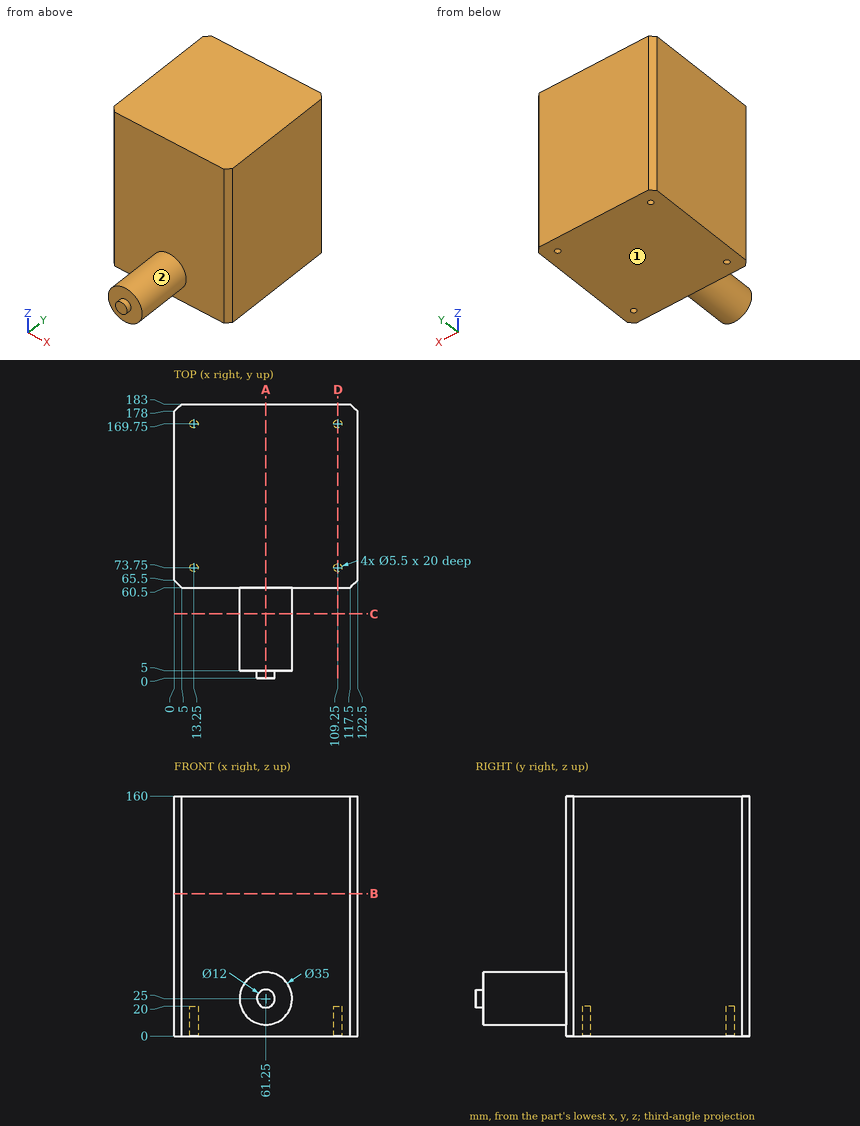
Can you work these out from the drawing? Everything is in mm from the part's minimum corner. A direction names the side the tool comes from. Round coordinates to 2 decimals unless told otherwise and drop trailing zeros. Loops run counter-clockwise (first coordinate to the right, second up) from the corner with the lowest first, then second, coordinate; pieces in that order, holes last. Notation, with made-up numbers: (31, -32) -> (55, -32) arc R29 cw to (55, -2) -> close; hole circle Ø7 at (9, -34). An arc over 180 degrees is marked (long way). Use CSV: the item, a comma, the result in double quotes.
(1) Suppose I cut it at C-C on y = 43. Write out the boundary of the cut face in (x, z), plus the area to 3 significant figures.
Return value:
outline,"circle Ø35 at (61.25, 25)"
area,"962 mm²"
(2) If I drill on probe 1 along Y at (x, z) = (13.25, 5.5); probe 2 along X at (y, z) = (169.75, 7.5); probe 3 along Y at (x, z) = (100.5, 55.5), over which ranges is the centre line in solid material (lowest first)? Write a range as [from, to].
Return value:
probe 1,"y = [60.5, 71], [76.5, 167], [172.5, 183]"
probe 2,"x = [0, 10.5], [16, 106.5], [112, 122.5]"
probe 3,"y = [60.5, 183]"
(3) For the marked faces 1 and 2, which set-ups out of +Z, -Z, +X, -X, +Y, -Y let a thin tool reach every point of the face, with its end or its side?
Return value:
face 1,"-Z, +X, -X, +Y, -Y"
face 2,"-Y"
(4) Suppose I cut it at B-B on z = 95. Write out the boundary of the cut face in (x, y).
Return value:
outline,"(0, 65.5) -> (5, 60.5) -> (117.5, 60.5) -> (122.5, 65.5) -> (122.5, 178) -> (117.5, 183) -> (5, 183) -> (0, 178) -> close"
(5) Will these pins go through, and if not, where does the flat tip stop? pin 1 Ø4.5 at (x, y) = (109.25, 169.75) entering from -Z; pin 2 Ø6 at (x, y) = (58.5, 42.5) entering from -Z; pin 3 Ø4.5 at (x, y) = (109.5, 75) entering from -Z; pin 4 Ø12 at (x, z) = (88.5, 62) entering from -Y.
Return value:
pin 1,"stops at z = 20"
pin 2,"stops at z = 7.5"
pin 3,"stops at z = 0"
pin 4,"stops at y = 60.5"
(6) Suppose I cut it at A-A on x = 61.25. Write out the boundary of the cut face in (y, z).
Return value:
outline,"(0, 19) -> (5, 19) -> (5, 7.5) -> (60.5, 7.5) -> (60.5, 0) -> (183, 0) -> (183, 160) -> (60.5, 160) -> (60.5, 42.5) -> (5, 42.5) -> (5, 31) -> (0, 31) -> close"
(7) Suppose I cut it at D-D on x = 109.25. Write out the boundary of the cut face in (y, z), plus the area to 3 significant figures.
Return value:
outline,"(60.5, 0) -> (71, 0) -> (71, 20) -> (76.5, 20) -> (76.5, 0) -> (167, 0) -> (167, 20) -> (172.5, 20) -> (172.5, 0) -> (183, 0) -> (183, 160) -> (60.5, 160) -> close"
area,"19,400 mm²"
